For this review, take the finished solid that the model builds, in its own axes (mm). Round coordinates to 2 decimals unless told otherwise and drop trailing zeros. Order: outer loops, then holes, each group sorted by start corner. A loop starts at its lowest first (then second) coordinate and runs counter-clockwise, first axis right, second up.
Autodesk Inventor part; units mm, degrees
ref_plane "YZ Plane" through (0, 0, 0) normal (1, 0, 0) x (0, 1, 0)
ref_plane "XZ Plane" through (0, 0, 0) normal (0, 1, 0) x (-1, 0, 0)
ref_plane "XY Plane" through (0, 0, 0) normal (0, 0, 1) x (1, 0, 0)
sketch "Sketch2" plane through (0, 0, 0) normal (0, 0, 1) x (1, 0, 0)
  line L0 (0, 0) -> (44.45, 0)
  line L1 (44.45, 0) -> (44.45, 90)
  line L2 (0, 90) -> (0, 0)
  arc A0 (44.45, 90) -> (0, 90) centre (22.225, 70.3025) ccw
  dimension "d3" = 44.45
  dimension "d4" = 100
  dimension "d5" = 90
extrude "Extrusion1" add sketch "Sketch2" along normal blind 3.175
chamfer "Chamfer1" distance 2 angle 45 2 edges at (44.45, 90, 1.5875) (0, 90, 1.5875)
sketch "Sketch3" plane through (0, 0, 3.175) normal (0, 0, 1) x (1, 0, 0)
  line L0 (0, 88) -> (0, 0)
  line L1 (0, 0) -> (44.45, 0)
  point P0 (22.225, 80)
  point P1 (22.225, 0)
  dimension "d13" = 80
hole "Hole1" at (22.225, 80, 3.175) direction (0, 0, -1) diameter 17 end through all
fillet "Fillet1" radius 0.5 1 edges at (22.225, 88.5, 3.175)
sketch "Sketch4" plane through (0, 0, 3.175) normal (0, 0, 1) x (1, 0, 0)
  line L0 (0, 0) -> (44.45, 0)
  line L1 (0, 88) -> (0, 0)
  line L2 (44.45, 0) -> (44.45, 88)
  point P0 (11.1125, 10.7938)
  point P1 (33.325, 10.7938)
  dimension "d22" = 44.45
  dimension "d23" = 11.1125
  dimension "d24" = 11.125
hole "Hole2" at (11.1125, 10.7938, 3.175) at (33.325, 10.7938, 3.175) direction (0, 0, -1) diameter 4.2333 end through all
properties part number "platen_support"
Q1. Mouldability with a two-part tool opening along X and no side actions: class faces 1 (the face through (35.39, 11.25, 1.57)), 2 (the face through (22, 0, 2)), 3 (the face through (44.45, 43, 2)) as +X half, -X half, draft (parallel to the pull), parting line (faces both ways), or undercut.
Q2. Take a section at A-A, the plane y = 80. State the section outline as (x, z) points (3 decimals), plus the area to 3 significant figures.
Q3. Clearance check with a flat-ended pin moving along its axis: pin 1 (1 mm diameter, centred on x = 6.5, y = 29.5, fed in from -Z). State where the tip first meets the part, or that it passes through.
Q4. Take a section at B-B, the plane z = 2.1. Count the separate pieces of the cut face and the enclosed holes in it, plus the area to 3 significant figures.
Q5. Wall thickness on line 1 (X direction, y = 80, z = 2.1) (3 decimals); line 2 (Y direction, x = 22, z = 0.7); line 3 (Y direction, x = 34.5, z = 1.95): over which ranges is each line inside the solid? List them lowest first.
Working result:
1. face 1: undercut
1. face 2: draft
1. face 3: +X half
2. outline: (0, 0) - (13.725, 0) - (13.725, 2.675) arc R0.5 ccw to (13.225, 3.175) - (0, 3.175) - close; (30.725, 0) - (44.45, 0) - (44.45, 3.175) - (31.225, 3.175) arc R0.5 ccw to (30.725, 2.675) - close
2. area: 87.0 mm2
3. pin 1: stops at z = 0
4. separate pieces: 1
4. enclosed holes: 3
4. area: 4,050 mm2
5. line 1: x = 0 to 13.725, 30.725 to 44.45
5. line 2: y = 0 to 71.5, 88.5 to 100
5. line 3: y = 0 to 9.03, 12.55 to 97.34
